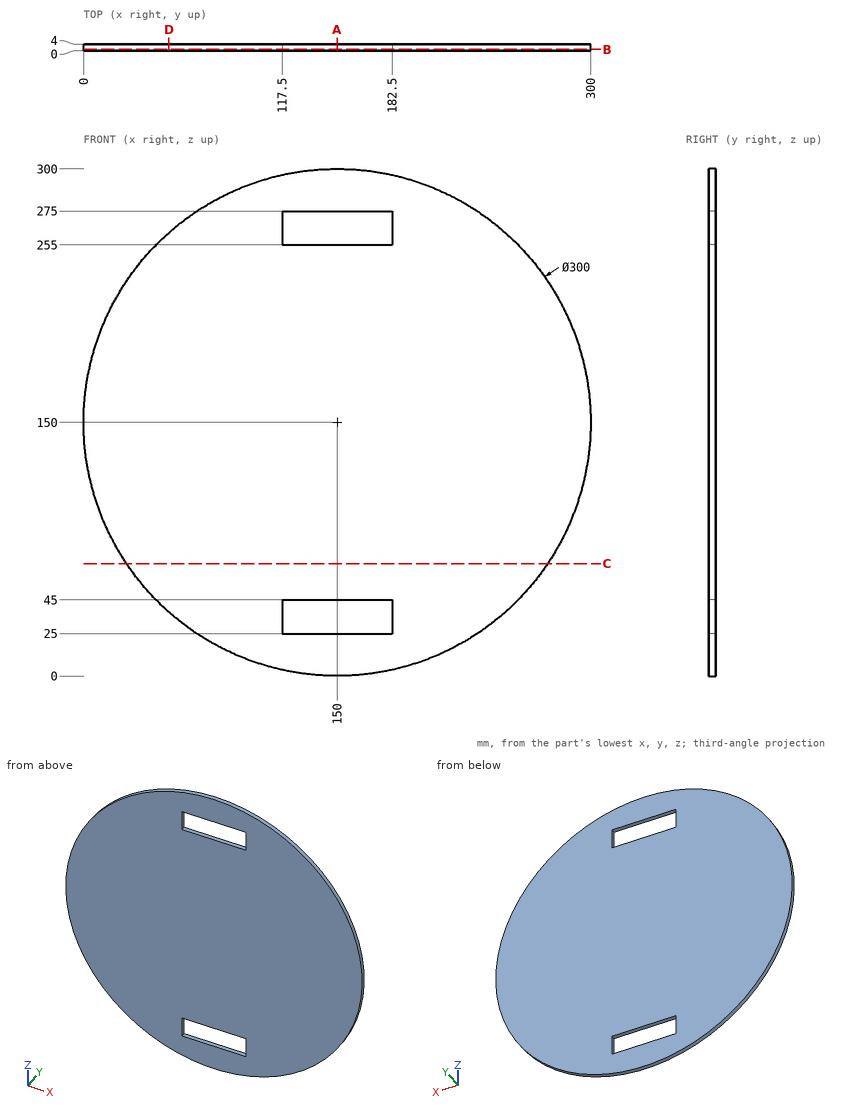
The drawing under review shows one solid part. Ordinate dimensions are in mm from its lowest x, y, z. Round coordinates to 2 decimals unless told otherwise and drop trailing zeros. Loops run counter-clockwise (first coordinate to the right, second up) from the corner with the lowest first, then second, coordinate; pieces in that order, holes last. Notation, with made-up numbers: (41, 79) - (54, 79) arc R11 cw to (54, 98) - close; hole circle Ø11 at (-30.5, -38). An arc over 180 degrees is marked (long way). One line per item, written item: value. Start each with the question number.
1) To check wall thickness, follow L1, parallel to Z at x = 123.5, y = 2.5; L2, parallel to X at y = 3.7, z = 259; L3, parallel to Z at x = 156.5, y = 3.1. State the ranges of each line that lie inside material, in increasing order. Write a range as from..to.
2) Consider section A-A on x = 150. Give the boundary of the cut face in (y, z).
3) Insertion check: pin 1 Ø1.2 at (x, y) = (161.5, 2.5) entering from +Z; pin 2 Ø2 at (y, z) = (1, 31) entering from -X; pin 3 Ø2 at (y, z) = (2, 38) entering from +X. Each pin has a flat end and moves straight along its axis. Give the tip position at first contact, or say it passes through.
4) Consider section D-D on x = 50.5. Give the boundary of the cut face in (y, z).
5) Consider section B-B on y = 0.8. Give the boundary of the cut face in (x, z).
6) Consider section C-C on z = 66.5. Give the boundary of the cut face in (x, y).
Reported:
1. L1: z = 2.36..25, 45..255, 275..297.64
1. L2: x = 46.95..117.5, 182.5..253.05
1. L3: z = 0.14..25, 45..255, 275..299.86
2. outline: (0, 0) - (4, 0) - (4, 25) - (0, 25) - close; (0, 45) - (4, 45) - (4, 255) - (0, 255) - close; (0, 275) - (4, 275) - (4, 300) - (0, 300) - close
3. pin 1: stops at z = 299.6
3. pin 2: stops at x = 57.39
3. pin 3: stops at x = 250.89
4. outline: (0, 37.75) - (4, 37.75) - (4, 262.25) - (0, 262.25) - close
5. outline: circle Ø300 at (150, 150); hole (117.5, 25) - (182.5, 25) - (182.5, 45) - (117.5, 45) - close; hole (117.5, 255) - (182.5, 255) - (182.5, 275) - (117.5, 275) - close
6. outline: (25.39, 0) - (274.61, 0) - (274.61, 4) - (25.39, 4) - close
